Source: CAD feature listing. Evaluate the final solid. Frame: model axes, mm. A direction names the side the tool comes from. Coordinates: 2 decimals unless noted, no trailing zeros. Order: outer loops, then holes, each group sorted by start corner. A loop starts at its lowest first (then second) coordinate and runs counter-clockwise, first axis right, second up. Notation, with made-up numbers: (78, 30) - (107, 30) arc R20 ccw to (107, 39) - close; hole circle Ø6 at (39, 36). An arc over 180 degrees is marked (long way). One line per question, with ' | ' between items. Start each with the question number.
(1) Contact query for flat-ended pins moving along their axis: P1, Ø12, axis at y = 17, z = 19, coming from the +X side; P2, Ø5, axis at x = -12.5, z = 34, coming from the -Y side; P3, Ø20.5, axis at x = 0, y = 4.5, coming from the -Z side; P4, Ø20.5, axis at x = -38.1, y = -19.05, coming from the +Z side. Output: stop coordinate, or through.
(2) Access query for faces 4 (the flat face through (10, 13, 12.7)), 5 (the cylindrical face through (31.756, 19.329, 6.439)), 6 (the cylindrical face through (-1.323, 10.074, 25.436)). Directions: +Z, -Z, +X, -X, +Y, -Y. A direction counts if a zero-diameter tool reaches every point of the face in a straight line with its end or side. Return the directions, or none.
(3) Section A-A (y = 19.05). Return the cut outline in (x, z).
(4) Section C-C (z = 5). Return the cut outline in (x, y).
(5) Draft query along Y for faces 1 (the cylindrical face through (-32.043, 20.957, 6.439)), 2 (the cylindrical face through (-2.75, -12.4, 17.82)), 3 (the flat face through (49.55, -0.44, 11.41)). Return one class per face: +Y half, -Y half, draft (parallel to the pull), parting line (faces both ways), or undercut.
(6) Line query: line 1 along Y through (x, z) = (-38.1, 9.25); line 2 along X through (y, z) = (-19, 7); line 3 along Y through (x, z) = (38.1, 10.25). Output: solid intervals per line, ascending.
(7) Section B-B (x = 38.1). Return the cut outline in (y, z), then the cut area to 3 significant figures.
from build123d import *

# Parameters (mm, degrees)
F0_W     = 101.6
F0_H     = 63.5
F1_DEPTH = 12.7
F2_R     = 6.35
F3_DEPTH = 12.701
F4_W     = 12.7
F4_H     = 25.4
F6_W     = 4.7343277841
F6_H     = 5.08
F6_W_2   = 2.54
F8_R     = 2.53999
F9_R     = 2.54
F10_SIZE = 2.54


# Not quite as in the source:
# - a fillet or chamfer is up to 0.001 mm smaller than in the source, because OpenCascade refuses the exact size


with BuildPart() as f1:
    # F0 (on Top) → F1 (new body)
    with BuildSketch(Plane.XY):
        Rectangle(F0_W, F0_H)
    extrude(amount=F1_DEPTH)

    # F2 (on face) → F3 (cut, through all)
    with BuildSketch(Plane.XY.offset(12.7)):
        with Locations((-38.1, 19.05)):
            Circle(F2_R)
        with Locations((38.1, 19.05)):
            Circle(F2_R)
        with Locations((38.1, -19.05)):
            Circle(F2_R)
        with Locations((-38.1, -19.05)):
            Circle(F2_R)
    extrude(amount=-F3_DEPTH, mode=Mode.SUBTRACT)

    # F4 (on Front) → F5 (revolve)
    with BuildSketch(Plane.XZ):
        with Locations((6.35, 25.4)):
            Rectangle(F4_W, F4_H)
    revolve(axis=Axis((0, 0, 25.4), (0, 0, 1)))

    # F6 (on Front) → F7 (revolve, cut)
    with BuildSketch(Plane.XZ):
        with Locations((15.067163892, 25.4)):
            Rectangle(F6_W, F6_H)
        with Locations((11.43, 25.4)):
            Rectangle(F6_W_2, F6_H)
    revolve(axis=Axis((0, 0, 12.7), (0, 0, 1)), mode=Mode.SUBTRACT)

    # F8 (radius 2.54 in the source; OpenCascade refuses exactly that, so slightly less here)
    f8_edges = [f1.edges().sort_by_distance(p)[0] for p in [
        (-12.7, 0, 12.7),
        (-12.7, 0, 22.86),
    ]]
    fillet(f8_edges, radius=F8_R)

    # F9
    f9_edges = [f1.edges().sort_by_distance(p)[0] for p in [
        (-12.7, 0, 38.1),
    ]]
    fillet(f9_edges, radius=F9_R)

    # F10
    f10_edges = [f1.edges().sort_by_distance(p)[0] for p in [
        (-50.8, 0, 12.7),
        (0, -31.75, 12.7),
        (0, 31.75, 12.7),
        (50.8, 0, 12.7),
    ]]
    chamfer(f10_edges, length=F10_SIZE)


solid = f1.part
Response values:
1) P1: stops at x = 6.35 | P2: stops at y = -7.83 | P3: stops at z = 0 | P4: stops at z = 12.7
2) face 4: +Z | face 5: +Z, -Z | face 6: none
3) outline: (-50.8, 0) - (-44.45, 0) - (-44.45, 12.7) - (-48.26, 12.7) - (-50.8, 10.16) - close; (-31.75, 0) - (31.75, 0) - (31.75, 12.7) - (-31.75, 12.7) - close; (44.45, 0) - (50.8, 0) - (50.8, 10.16) - (48.26, 12.7) - (44.45, 12.7) - close
4) outline: (-50.8, -31.75) - (50.8, -31.75) - (50.8, 31.75) - (-50.8, 31.75) - close; hole circle Ø12.7 at (-38.1, -19.05); hole circle Ø12.7 at (-38.1, 19.05); hole circle Ø12.7 at (38.1, -19.05); hole circle Ø12.7 at (38.1, 19.05)
5) face 1: undercut | face 2: parting line | face 3: draft
6) line 1: y = -31.75 to -25.4, -12.7 to 12.7, 25.4 to 31.75 | line 2: x = -50.8 to -44.45, -31.75 to 31.75, 44.45 to 50.8 | line 3: y = -31.66 to -25.4, -12.7 to 12.7, 25.4 to 31.66
7) outline: (-31.75, 0) - (-25.4, 0) - (-25.4, 12.7) - (-29.21, 12.7) - (-31.75, 10.16) - close; (-12.7, 0) - (12.7, 0) - (12.7, 12.7) - (-12.7, 12.7) - close; (25.4, 0) - (31.75, 0) - (31.75, 10.16) - (29.21, 12.7) - (25.4, 12.7) - close | area: 477 mm²
